Build history of the part. All positions in model axes, mm. Face numbers are marked on the shaded views. A direction names the side the tool comes from. Round coordinates to 2 decimals unless told otherwise and drop trailing zeros. Write each loop counter-clockwise with the first axis right and the second up, starting at its lowest first coordinate (ties: lowest second). Pieces come first, ordered by that corner, then holes.
Item 1: Wall check: probe 1 along Y at (x, z) = (-13.75, -5); probe 2 along X at (y, z) = (0.5, -10.5); probe 3 along X at (y, z) = (22, -9.5). Give the ranges that are in metal, low to high.
Item 2: Band-saw the part on A-A, the plane x = -30.5. Write the cut outline in (y, z) (3 decimals).
Item 3: Drop flat-ended pins along their axis: pin 1 Ø2 at (y, z) = (3.5, -14) entering from +X; pin 2 Ø6 at (y, z) = (1, 13.5) entering from +X; pin 3 Ø12 at (x, y) = (-22, 6) entering from -Z; pin 4 Ø6 at (y, z) = (0, -1.5) entering from -X. Give the stop position or say it passes through.
Item 4: 3-axis set-ups, long thin cutter, end or side, ignore diameter. For the marked faces 1, 2, 3 and 4: which of +Z, -Z, +X, -X, +Y, -Y reach the whole face in a straight line?
Item 5: Mould opens along Y. For the marked faces 5, 6, 7 and 8 say: +Y half, -Y half, draft (parallel to the pull), parting line (faces both ways), or undercut.
Item 6: Band-saw the part on B-B, the plane z = 1. Write the cut outline in (x, y), then the cut area to 3 significant figures.
Item 7: Band-saw the part on D-D, the plane y = 9. Write the cut outline in (x, z), then the cut area to 3 significant figures.
Item 8: Band-saw the part on C-C, the plane x = -16.5. Write the cut outline in (y, z) (3 decimals), then the cut area to 3 significant figures.
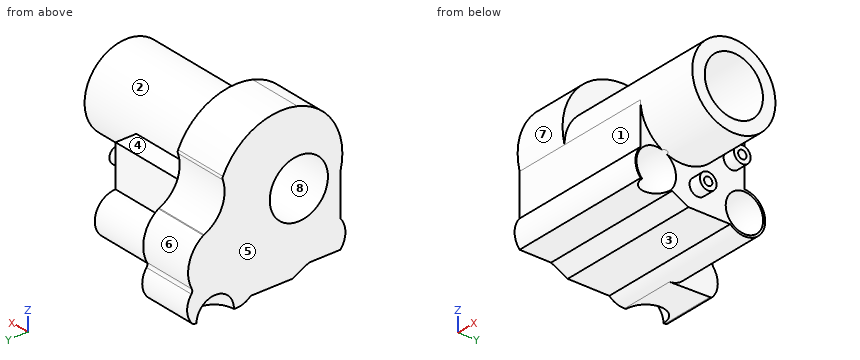
```python
from build123d import *

# Parameters (mm, degrees)
SKETCH1_R           = 10
BOSS_EXTRUDE1_DEPTH = 50
BOSS_EXTRUDE3_DEPTH = 35
SKETCH8_R           = 2
SKETCH8_R_2         = 1
BOSS_EXTRUDE4_DEPTH = 3
BOSS_EXTRUDE6_DEPTH = 13
FILLET1_R           = 1
FILLET2_R           = 1
SKETCH2_R           = 7
CUT_EXTRUDE2_DEPTH  = 61.180591


with BuildPart() as part:
    # Sketch1 → Boss-Extrude1 (new body)
    with BuildSketch(Plane(origin=(0, 0, 0), x_dir=(0, 0, -1), z_dir=(1, 0, 0))):
        Circle(SKETCH1_R)
    extrude(amount=-BOSS_EXTRUDE1_DEPTH)

    # Sketch3 → Boss-Extrude3 (add)
    with BuildSketch(Plane(origin=(-50, 0, 0), x_dir=(0, 0, -1), z_dir=(1, 0, 0))):
        with BuildLine():
            Line((0, 10), (0, 15))
            Line((0, 15), (10, 15))
            ThreePointArc((10, 15), (16.842071907, 19.648308412), (18.642708436, 11.574992664))
            Line((18.642708436, 11.574992664), (18.642708436, 1.574992664))
            Line((18.642708436, 1.574992664), (16.642708436, -2.425007336))
            Line((16.642708436, -2.425007336), (16.642708436, -9.997750449))
            ThreePointArc((16.642708436, -9.997750449), (13.321760405, -11.198307119), (10, -10))
            Line((10, -10), (0, -10))
            Line((0, -10), (0, 10))
        make_face()
    extrude(amount=BOSS_EXTRUDE3_DEPTH)

    # Sketch6 → Cut-Revolve1 (revolve, cut)
    with BuildSketch(Plane(origin=(-15, 0, 0), x_dir=(0, 0, -1), z_dir=(1, 0, 0))):
        with BuildLine():
            Line((13.321760405, -1.448307119), (13.321760405, -10.948307119))
            ThreePointArc((13.321760405, -10.948307119), (18.071760405, -6.198307119), (13.321760405, -1.448307119))
        make_face()
    revolve(axis=Axis((-15, -1.448307119, -13.321760405), (0, -1, 0)), mode=Mode.SUBTRACT)

    # Sketch7 → Cut-Revolve2 (revolve, cut)
    with BuildSketch(Plane(origin=(-15, 0, 0), x_dir=(0, 0, -1), z_dir=(1, 0, 0))):
        with BuildLine():
            Line((15, 10.5), (15, 19.5))
            ThreePointArc((15, 19.5), (19.5, 15), (15, 10.5))
        make_face()
    revolve(axis=Axis((-15, 10.5, -15), (0, 1, 0)), mode=Mode.SUBTRACT)

    # Sketch8 → Boss-Extrude4 (add)
    # profile 1 of 2: a face of its own
    with BuildSketch(Plane(origin=(-15, 0, 0), x_dir=(0, 0, -1), z_dir=(1, 0, 0))):
        with Locations(Location((13.642708436, 3.801692881, 0), (0, 0, 180))):
            Circle(SKETCH8_R)
        with Locations((13.642708436, 3.801692881)):
            Circle(SKETCH8_R_2, mode=Mode.SUBTRACT)
    # profile 2 of 2: a face of its own
    with BuildSketch(Plane(origin=(-15, 0, 0), x_dir=(0, 0, -1), z_dir=(1, 0, 0))):
        with Locations(Location((5, 12, 0), (0, 0, 180))):
            Circle(SKETCH8_R)
        with Locations((5, 12)):
            Circle(SKETCH8_R_2, mode=Mode.SUBTRACT)
    extrude(amount=BOSS_EXTRUDE4_DEPTH)

    # Sketch10 → Boss-Extrude6 (add)
    with BuildSketch(Plane.ZY.offset(50)):
        with BuildLine():
            Line((-19.714603594, 25.400073987), (-19.992475161, 15.274211174))
            ThreePointArc((-19.992475161, 15.274211174), (-14.862842799, 19.998118436), (-10, 15))
            Line((-10, 15), (0, 15))
            Line((0, 15), (0, 10))
            ThreePointArc((0, 10), (10, 0), (0, -10))
            ThreePointArc((0, -10), (10.951955319, -8.476456548), (17.618849286, 0.345053233))
            ThreePointArc((17.618849286, 0.345053233), (16.545732573, 11.017476726), (8.77988791, 18.416386062))
            ThreePointArc((8.77988791, 18.416386062), (2.657537615, 18.500996178), (-1.611789409, 22.889979975))
            ThreePointArc((-1.611789409, 22.889979975), (-6.607805104, 26.429776463), (-12.643535782, 25.400073987))
            ThreePointArc((-12.643535782, 25.400073987), (-16.179069688, 26.864540081), (-19.714603594, 25.400073987))
        make_face()
    extrude(amount=-BOSS_EXTRUDE6_DEPTH)

    # Fillet1
    fillet1_edges = [part.edges().sort_by_distance(p)[0] for p in [
        (-43.5, 25.400073987, -12.643535782),
        (-43.5, 22.889979975, -1.611789409),
        (-43.5, 18.416386062, 8.77988791),
    ]]
    fillet(fillet1_edges, radius=FILLET1_R)

    # Fillet2
    fillet2_edges = [part.edges().sort_by_distance(p)[0] for p in [
        (-43.5, 25.400073987, -19.714603594),
    ]]
    fillet(fillet2_edges, radius=FILLET2_R)

    # Sketch11 → Cut-Revolve3 (revolve, cut)
    with BuildSketch(Plane(origin=(0, 0.559709606, -20.396267082), x_dir=(-1, 0, 0), z_dir=(0, 0.02743144017102401, -0.999623687239425))):
        with BuildLine():
            Line((50, 24.072659381), (50, 15.072659381))
            ThreePointArc((50, 15.072659381), (45.5, 19.572659381), (50, 24.072659381))
        make_face()
    revolve(axis=Axis((-50, 24.623310138, -19.735919367), (0, -0.9996236872394249, -0.027431440171024075)), mode=Mode.SUBTRACT)

    # Sketch2 → Cut-Extrude2 (cut, through all)
    with BuildSketch(Plane(origin=(0, 0, 0), x_dir=(0, 0, -1), z_dir=(1, 0, 0))):
        Circle(SKETCH2_R)
    extrude(amount=-CUT_EXTRUDE2_DEPTH, mode=Mode.SUBTRACT)


solid = part.part
```
Results:
1. probe 1: y = -8.66 to -4.9, 4.9 to 8.66, 10 to 11, 13 to 14
1. probe 2: x = -50 to -15
1. probe 3: x = -50 to -37
2. outline: (-10, -10) arc R5.198 ccw to (-9.998, -16.643) - (-2.425, -16.643) - (1.575, -18.643) - (11.575, -18.643) arc R5 ccw (long way) to (15, -10) - (15, 0) - (10, 0) arc R10 ccw to (-10, 0) - close; hole circle Ø14 at (0, 0)
3. pin 1: stops at x = -12
3. pin 2: stops at x = -37
3. pin 3: stops at z = -19
3. pin 4: passes through
4. face 1: +X, -X, -Y
4. face 2: +X
4. face 3: -Z, +X, -X, -Y
4. face 4: +Z, +X, +Y
5. face 5: draft
5. face 6: +Y half
5. face 7: -Y half
5. face 8: undercut
6. outline: (-50, -10.22) - (-37, -10.22) - (-37, -9.95) - (0, -9.95) - (0, -6.93) - (-50, -6.93) - close; (-50, 6.93) - (0, 6.93) - (0, 9.95) - (-37, 9.95) - (-37, 19.46) - (-50, 19.46) - close
6. area: 429 mm2
7. outline: (-50, -18.64) - (-15, -18.64) - (-15, -4.36) - (0, -4.36) - (0, 4.36) - (-37, 4.36) - (-37, 17.36) - (-50, 17.36) - close
7. area: 1,100 mm2
8. outline: (-10, -10) arc R5.198 ccw to (-9.998, -16.643) - (-9.245, -16.643) arc R4.507 cw (long way) to (-3.151, -16.643) - (-2.425, -16.643) - (1.575, -18.643) - (11.575, -18.643) arc R5 ccw (long way) to (15, -10) - (15, 0) - (10, 0) arc R10 ccw to (-10, 0) - close; hole circle Ø14 at (0, 0); hole circle Ø8.485 at (15, -15)
8. area: 383 mm2
